For this review, use the dimensioned drawing (mm, ordinates from the lowest corner) and the shaded views. A direction names the side the tool comes from. Round coordinates to 2 decimals unless told otherwise and drop trailing zeros. Write each loop counter-clockwise with the first axis right and the second up, starting at its lowest first coordinate (ties: lowest second). Pieces come first, ordered by that corner, then holes. Notation, with made-up numbers: (-8.5, 47.5) -> (47.5, 47.5) arc R34 ccw to (47.5, 86.5) -> close; hole circle Ø9 at (53.25, 23). An arc over 180 degrees is marked (long way). Answer in a Markdown table with one row per item. Add a question column.
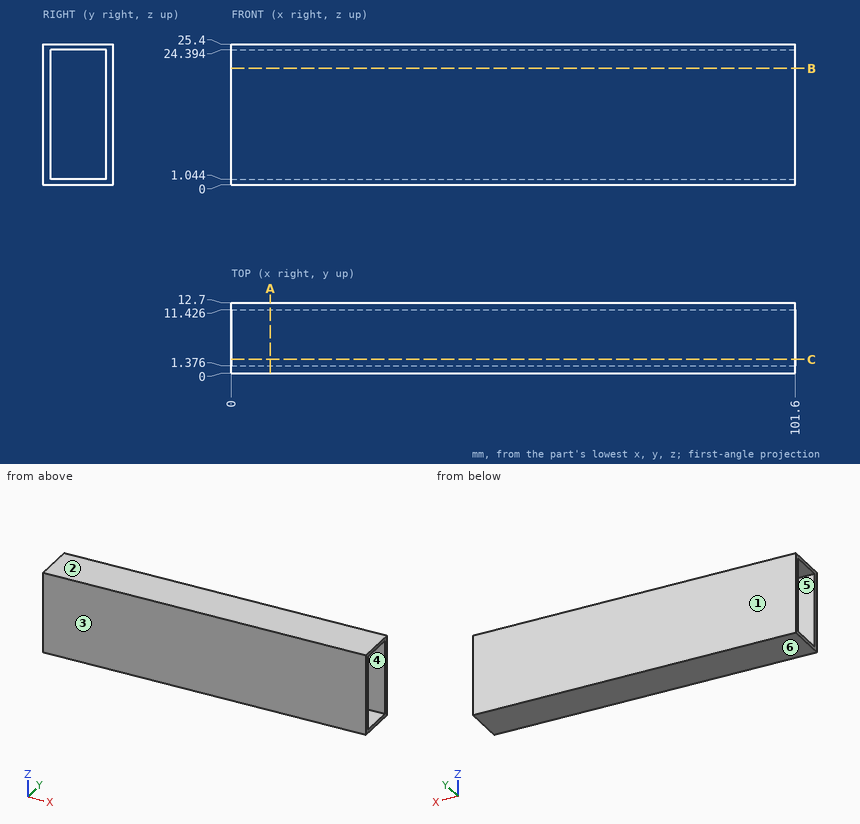
1. The part is to be moulded in two halves that separate along Y. For the marked faces 1, 2, 3 and 4, say which applies: pulls with the +Y half, pulls with the -Y half, needs draft (parallel to the pull), parting line crosses it, or undercut.
2. Tool access review of the marked faces 5 and 6: name each direction out of +Z, -Z, +X, -X, +Y, -Y from which nothing blocks a thin tool from reaching the whole face with its end or side.
3. Clearance check with a flat-ended pin moving along its axis: pin 1 Ø3 at (x, y) = (75.5, 2) entering from -Z. State where the tip first meets the part, or that it passes through.
4. We need section C-C (y = 2.5). Write out the cut boundary in (x, z) (1 decimal).
5. We need section A-A (x = 7). Write out the cut boundary in (y, z) (1 decimal).
6. We need section B-B (z = 21). Write out the cut boundary in (x, y).
7. For L1, parallel to Y at x = 77.5, z = 5.25; L2, parallel to Z at x = 93, y = 10.25 (1 decimal), list the stretches that pass through material, from the lowest coordinate up. Write a range as [from, to].
Response:
| question | item | result |
|---|---|---|
| 1 | face 1 | pulls with the +Y half |
| 1 | face 2 | needs draft |
| 1 | face 3 | pulls with the -Y half |
| 1 | face 4 | undercut |
| 2 | face 5 | +X, -X |
| 2 | face 6 | -Z, +X, -X, +Y, -Y |
| 3 | pin 1 | z = 0 |
| 4 | outline | (0, 0) -> (101.6, 0) -> (101.6, 1) -> (0, 1) -> close; (0, 24.4) -> (101.6, 24.4) -> (101.6, 25.4) -> (0, 25.4) -> close |
| 5 | outline | (0, 0) -> (12.7, 0) -> (12.7, 25.4) -> (0, 25.4) -> close; hole (1.4, 1) -> (11.4, 1) -> (11.4, 24.4) -> (1.4, 24.4) -> close |
| 6 | outline | (0, 0) -> (101.6, 0) -> (101.6, 1.38) -> (0, 1.38) -> close; (0, 11.43) -> (101.6, 11.43) -> (101.6, 12.7) -> (0, 12.7) -> close |
| 7 | L1 | [0, 1.38], [11.43, 12.7] |
| 7 | L2 | [0, 1], [24.4, 25.4] |
